For this review, take the finished solid that the model builds, in its own axes (mm). A direction names the side the tool comes from. Round coordinates to 2 decimals unless told otherwise and drop trailing zeros. Write each loop counter-clockwise with the first axis right and the second up, starting at its lowest first coordinate (ties: lowest second). Pieces come first, ordered by that corner, then holes. Notation, with made-up numbers: (-9.5, -7) -> (10.5, -7) arc R28 ccw to (10.5, 17) -> close; hole circle Ø11 at (39.5, 74). An arc over 180 degrees is marked (long way). Answer in a Markdown table with one row per item. Add a question column.
```python
from build123d import *

# Parameters (mm, degrees)
F3_R     = 3.2
F4_DEPTH = 9.907
F5_R     = 9.16
F5_R_2   = 7.1798
F5_R_3   = 6.1798
F5_R_4   = 4.2
F6_DEPTH = 1


with BuildPart() as f1:
    # F0 (on Front) → F1 (revolve)
    with BuildSketch(Plane.XZ):
        Polygon((0, 0), (0, 4.953), (-10.16, 4.953), (-10.16, 1.6510004181), (-7.62, 1.6510004181), (-7.62, 0), align=None)
        with BuildLine():
            Line((-7.62, 1.6510004181), (-10.16, 1.6510004181))
            add(Edge.make_bspline(
                [(-7.62, 0), (-7.62, 0.8255002091), (-8.89, 1.6510004181), (-10.16, 1.6510004181)],
                knots=[0, 0, 0, 0, 3.0294227801, 3.0294227801, 3.0294227801, 3.0294227801], degree=3))
            Line((-7.62, 0), (-7.62, 1.6510004181))
        make_face()
    revolve(axis=Axis((0, 0, 12.7), (0, 0, 1)))

    # F2: F1 across plane


with BuildPart() as f1_1:
    add(f1.part)
    add(f1.part.mirror(Plane.XY))

    # F3 (on face) → F4 (cut, through all)
    with BuildSketch(Plane.XY.offset(4.953)):
        Circle(F3_R)
    extrude(amount=-F4_DEPTH, mode=Mode.SUBTRACT)

    # F5 (on face) → F6 (cut)
    with BuildSketch(Plane(origin=(0, 0, -4.953), x_dir=(1, 0, 0), z_dir=(0, 0, -1))):
        Circle(F5_R)
        Circle(F5_R_2, mode=Mode.SUBTRACT)
        Circle(F5_R_3)
        Circle(F5_R_4, mode=Mode.SUBTRACT)
    extrude(amount=-F6_DEPTH, mode=Mode.SUBTRACT)


solid = f1_1.part
```
1. For L1, parallel to Y at x = 0, z = -2.25; L2, parallel to Z at x = -1, y = -5.75; L3, parallel to Y at x = 0, z = -0.25, list the stretches that pass through material, from the lowest coordinate up. Write a range as [from, to].
2. The part is to be moulded in two halves that separate along X. For faces 1 (the cylindrical face through (-4.904, 3.76, -4.46)), 2 (the flat face through (-5, -8, -4.953)), 3 (the cylindrical face through (1.323, -10.074, 3.279)), say which applies: pulls with the +X half, pulls with the -X half, needs draft (parallel to the pull), parting line crosses it, or undercut.
3. We need section A-A (z = 2.5). Write out the cut boundary in (x, y).
4. Tool access review of faces 4 (the flat face through (-2.4, -2.4, 4.953)), 5 (the cylindrical face through (4.006, -1.262, -4.46)): name each direction out of +Z, -Z, +X, -X, +Y, -Y from which nothing blocks a thin tool from reaching the whole face with its end or side.
5. Clearance check with flat-ended pins moving along their axes: pin 1 Ø4 at (y, z) = (-3, 3.5) entering from -X; pin 2 Ø3 at (y, z) = (7, 3.5) entering from +X; pin 3 Ø1.5 at (y, z) = (-6.5, 3) entering from +X. State where each tip first meets the part, or that it passes through.
Response:
| question | item | result |
|---|---|---|
| 1 | L1 | [-10.16, -3.2], [3.2, 10.16] |
| 1 | L2 | [-3.95, 4.95] |
| 1 | L3 | [-7.66, -3.2], [3.2, 7.66] |
| 2 | face 1 | undercut |
| 2 | face 2 | needs draft |
| 2 | face 3 | parting line crosses it |
| 3 | outline | circle Ø20.32 at (0, 0); hole circle Ø6.4 at (0, 0) |
| 4 | face 4 | +Z, +X, -X, +Y, -Y |
| 4 | face 5 | -Z |
| 5 | pin 1 | x = -10.11 |
| 5 | pin 2 | x = 8.54 |
| 5 | pin 3 | x = 8.38 |
